The model under review builds one solid part; all positions refer to its coordinate system, in mm. Face numbers are marked on the shaded views. Round coordinates to 2 decimals unless told otherwise and drop trailing zeros. Loops run counter-clockwise (first coordinate to the right, second up) from the corner with the lowest first, then second, coordinate; pieces in that order, holes last. Notation, with made-up numbers: M -35,77.5 L 10,77.5 A17 cw 10,83.5 Z; hole C 52.5,57 d1. An arc over 180 degrees is marked long. Answer in a Markdown table with one row per item. Add a question column.
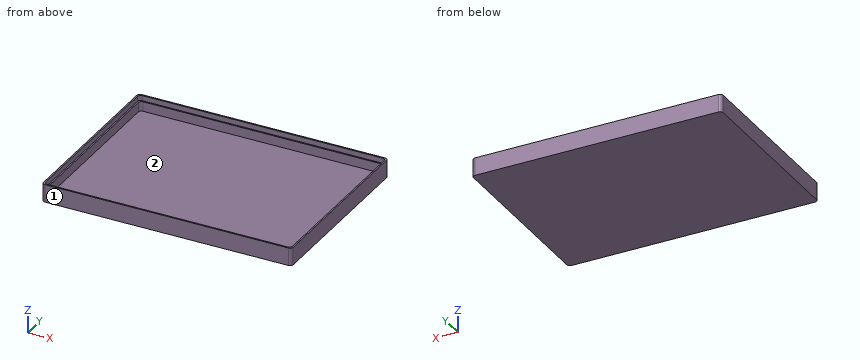
from build123d import *

# Parameters (mm, degrees)
F0_W     = 165
F0_H     = 119.8
F1_DEPTH = 10
F2_T     = 2
F3_W     = 167
F3_H     = 121.8
F4_DEPTH = 3.5
F5_R     = 2


with BuildPart() as f1:
    # F0 (on Top) → F1 (new body)
    with BuildSketch(Plane.XY):
        Rectangle(F0_W, F0_H)
    extrude(amount=F1_DEPTH)

    # F2
    f2_openings = [f1.faces().sort_by_distance(p)[0] for p in [
        (0, 0, 10),
    ]]
    offset(amount=F2_T, openings=f2_openings, kind=Kind.INTERSECTION)

    # F3 (on face) → F4 (cut)
    with BuildSketch(Plane.XY.offset(10)):
        Rectangle(F3_W, F3_H)
    extrude(amount=-F4_DEPTH, mode=Mode.SUBTRACT)

    # F5
    f5_edges = [f1.edges().sort_by_distance(p)[0] for p in [
        (-82.5, -59.9, 3.25),
        (82.5, -59.9, 3.25),
        (82.5, 59.9, 3.25),
        (-82.5, 59.9, 3.25),
        (-83.5, 60.9, 8.25),
        (-84.5, 61.9, 4),
        (83.5, 60.9, 8.25),
        (84.5, 61.9, 4),
        (-84.5, -61.9, 4),
        (-83.5, -60.9, 8.25),
        (84.5, -61.9, 4),
        (83.5, -60.9, 8.25),
    ]]
    fillet(f5_edges, radius=F5_R)


solid = f1.part
1. Take a section at B-B, the plane y = -0.5. State the section outline as (x, z) points, and give its area (3 significant figures).
2. For pin 1 Ø1.5 at (x, y) = (-44, 47) entering from +Z, flat-tipped, find the tip position at first contact; note if it passes through.
3. Mouldability with a two-part tool opening along X and no side actions: class the marked faces 1 and 2 as released by +X, released by -X, zero draft, split by the parting line, or undercut.
4. Take a section at C-C, the plane x = 1. State the section outline as (y, z) points, and give its area (3 significant figures).
5. To check wall thickness, follow probe 1 along Y at (x, z) = (-15, 7); probe 2 along Y at (x, z) = (13, 3.5); probe 3 along X at (y, z) = (-7.5, 5.25). State the ranges of each line that lie inside material, in increasing order.
6. Take a section at A-A, the plane z = 8.25. State the section outline as (x, y) points.
Check sheet entries:
| question | item | result |
|---|---|---|
| 1 | outline | M -84.5,-2 L 84.5,-2 L 84.5,10 L 83.5,10 L 83.5,6.5 L 82.5,6.5 L 82.5,0 L -82.5,0 L -82.5,6.5 L -83.5,6.5 L -83.5,10 L -84.5,10 Z |
| 1 | area | 371 mm^2 |
| 2 | pin 1 | stops at z = 0 |
| 3 | face 1 | zero draft |
| 3 | face 2 | undercut |
| 4 | outline | M -61.9,-2 L 61.9,-2 L 61.9,10 L 60.9,10 L 60.9,6.5 L 59.9,6.5 L 59.9,0 L -59.9,0 L -59.9,6.5 L -60.9,6.5 L -60.9,10 L -61.9,10 Z |
| 4 | area | 281 mm^2 |
| 5 | probe 1 | y = -61.9 to -60.9, 60.9 to 61.9 |
| 5 | probe 2 | y = -61.9 to -59.9, 59.9 to 61.9 |
| 5 | probe 3 | x = -84.5 to -82.5, 82.5 to 84.5 |
| 6 | outline | M -84.5,-59.9 A2 ccw -82.5,-61.9 L 82.5,-61.9 A2 ccw 84.5,-59.9 L 84.5,59.9 A2 ccw 82.5,61.9 L -82.5,61.9 A2 ccw -84.5,59.9 Z; hole M -83.5,-58.9 A2 ccw -81.5,-60.9 L 81.5,-60.9 A2 ccw 83.5,-58.9 L 83.5,58.9 A2 ccw 81.5,60.9 L -81.5,60.9 A2 ccw -83.5,58.9 Z |
